Here's how the part is built. I have some questions about the finished solid (model axes, mm). Face numbers are marked on the shaded views. A direction names the side the tool comes from. Coordinates: 2 decimals unless noted, no trailing zeros. Order: outer loops, then holes, each group sorted by start corner. A loop starts at its lowest first (then second) coordinate and runs counter-clockwise, first axis right, second up.
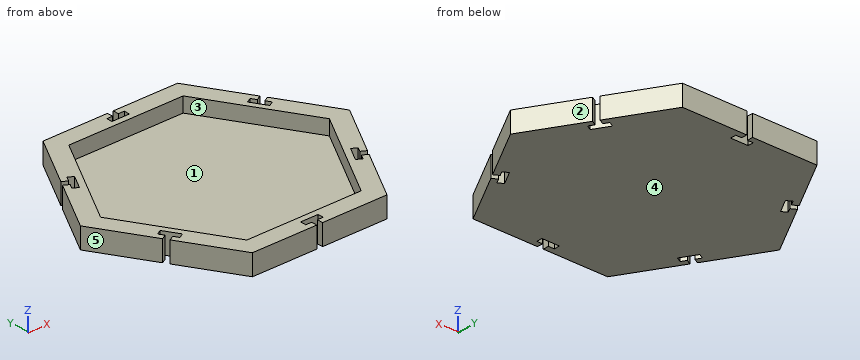
```python
from build123d import *

# Parameters (mm, degrees)
F1_DEPTH = 2
F3_DEPTH = 5


with BuildPart() as f1:
    # F0 (on Top) → F1 (new body)
    with BuildSketch(Plane.XY):
        Polygon((-24.740927, -24.347703), (-13.693921, -43.481678), (8.400089, -43.481678), (8.400089, -41.481678), (6.400089, -41.481678), (6.400089, -39.481678), (12.400089, -39.481678), (12.400089, -41.481678), (10.400089, -41.481678), (10.400089, -43.481678), (32.4941, -43.481678), (43.541105, -24.347703), (41.809055, -23.347703), (40.809055, -25.079754), (39.077004, -24.079754), (42.077004, -18.883602), (43.809055, -19.883602), (42.809055, -21.615652), (44.541105, -22.615652), (55.588111, -3.481678), (44.541105, 15.652297), (42.809055, 14.652297), (43.809055, 12.920246), (42.077004, 11.920246), (39.077004, 17.116398), (40.809055, 18.116398), (41.809055, 16.384348), (43.541105, 17.384348), (32.4941, 36.518322), (10.400089, 36.518322), (10.400089, 34.518322), (12.400089, 34.518322), (12.400089, 32.518322), (6.400089, 32.518322), (6.400089, 34.518322), (8.400089, 34.518322), (8.400089, 36.518322), (-13.693921, 36.518322), (-24.740927, 17.384348), (-23.008876, 16.384348), (-22.008876, 18.116398), (-20.276825, 17.116398), (-23.276825, 11.920246), (-25.008876, 12.920246), (-24.008876, 14.652297), (-25.740927, 15.652297), (-36.787932, -3.481678), (-25.740927, -22.615652), (-24.008876, -21.615652), (-25.008876, -19.883602), (-23.276825, -18.883602), (-20.276825, -24.079754), (-22.008876, -25.079754), (-23.008876, -23.347703), align=None)
    extrude(amount=F1_DEPTH)

    # F2 (on face) → F3 (join)
    with BuildSketch(Plane.XY.offset(2)):
        Polygon((-25.740927, -22.615652), (-24.008876, -21.615652), (-25.008876, -19.883602), (-23.276825, -18.883602), (-20.276825, -24.079754), (-22.008876, -25.079754), (-23.008876, -23.347703), (-24.740927, -24.347703), (-13.693921, -43.481678), (8.400089, -43.481678), (8.400089, -41.481678), (6.400089, -41.481678), (6.400089, -39.481678), (12.400089, -39.481678), (12.400089, -41.481678), (10.400089, -41.481678), (10.400089, -43.481678), (32.4941, -43.481678), (43.541105, -24.347703), (41.809055, -23.347703), (40.809055, -25.079754), (39.077004, -24.079754), (42.077004, -18.883602), (43.809055, -19.883602), (42.809055, -21.615652), (44.541105, -22.615652), (55.588111, -3.481678), (44.541105, 15.652297), (42.809055, 14.652297), (43.809055, 12.920246), (42.077004, 11.920246), (39.077004, 17.116398), (40.809055, 18.116398), (41.809055, 16.384348), (43.541105, 17.384348), (32.4941, 36.518322), (10.400089, 36.518322), (10.400089, 34.518322), (12.400089, 34.518322), (12.400089, 32.518322), (6.400089, 32.518322), (6.400089, 34.518322), (8.400089, 34.518322), (8.400089, 36.518322), (-13.693921, 36.518322), (-24.740927, 17.384348), (-23.008876, 16.384348), (-22.008876, 18.116398), (-20.276825, 17.116398), (-23.276825, 11.920246), (-25.008876, 12.920246), (-24.008876, 14.652297), (-25.740927, 15.652297), (-36.787932, -3.481678), align=None)
        Polygon((-10.22982, -37.481678), (-29.859729, -3.481678), (-10.22982, 30.518322), (29.029998, 30.518322), (48.659908, -3.481678), (29.029998, -37.481678), align=None, mode=Mode.SUBTRACT)
    extrude(amount=F3_DEPTH)


solid = f1.part
```
Q1. If we section it at B-B on y = 8: Write out the boundary of the cut face in (x, z).
Q2. I need wall thicknesses on L1, parallel to X at y = -19, z = 1; L2, parallel to Y at x = -1, z = 3; L3, parallel to X at y = -20, z = 4.5. Which ranges of each line are inside material? Lowest first, please.
Q3. For the marked faces 1 and 2, which set-ups out of +Z, -Z, +X, -X, +Y, -Y let a thin tool reach every point of the face, with its end or its side?
Q4. Will these pins go through, and if not, where does the flat tip stop? pin 1 (8 mm diameter, centred on x = -26.5, y = 5.5, fed in from -Z); pin 2 (3 mm diameter, centred on x = -10.5, y = 3, fed in from +Z); pin 3 (2 mm diameter, centred on y = -40.5, z = 4.5, fed in from -X); pin 4 (0.6 mm diameter, centred on y = -42.5, z = 4.5, fed in from -X).
Q5. We'd pull the mould along X, two halves only. Please class the marked faces 3, 4 and 5: pulls with the +X half, pulls with the -X half, needs draft (parallel to the pull), parting line crosses it, or undercut.
Q6. If we section it at A-A on x = 15: Write out the boundary of the cut face in (y, z), then the cut area to 3 significant figures.
Reply:
1. outline: (-30.16, 0) - (48.96, 0) - (48.96, 7) - (42.03, 7) - (42.03, 2) - (-23.23, 2) - (-23.23, 7) - (-30.16, 7) - close
2. L1: x = -27.83 to -23.48, -23.21 to 42.01, 42.28 to 46.63
2. L2: y = -43.48 to -37.48, 30.52 to 36.52
2. L3: x = -27.25 to -24.94, -22.63 to -20.32, 39.12 to 41.43, 43.74 to 46.05
3. face 1: +Z
3. face 2: +Z, -Z, +X, +Y
4. pin 1: stops at z = 0
4. pin 2: stops at z = 2
4. pin 3: stops at x = -15.99
4. pin 4: stops at x = -14.43
5. face 3: undercut
5. face 4: needs draft
5. face 5: pulls with the -X half
6. outline: (-43.48, 0) - (36.52, 0) - (36.52, 7) - (30.52, 7) - (30.52, 2) - (-37.48, 2) - (-37.48, 7) - (-43.48, 7) - close
6. area: 220 mm2
